The model under review builds one solid part; all positions refer to its coordinate system, in mm. Round coordinates to 2 decimals unless told otherwise and drop trailing zeros. Loops run counter-clockwise (first coordinate to the right, second up) from the corner with the lowest first, then second, coordinate; pieces in that order, holes last. Notation, with made-up numbers: (45, -36) -> (78, -36) arc R15 ccw to (78, -29) -> close; hole circle Ø10 at (29, 80). An arc over 180 degrees is marked (long way). Use a Markdown table: item, result. Add a question column.
1) Consider section D-D on z = 303. Give the boundary of the cut face in (x, y).
2) Consider section B-B on z = 212. Give the boundary of the cut face in (x, y), plus the area to 3 significant figures.
3) Consider section A-A on z = 277. Give the boundary of the cut face in (x, y), plus the area to 3 significant figures.
4) Consider section C-C on x = 9.5. Give the boundary of the cut face in (y, z).
5) Insertion check: pin 1 (1 mm diameter, centred on x = -31, y = 77.5, fed in from +Z); pin 2 (0.9 mm diameter, centred on y = 77, z = 316.5, fed in from -X); pin 3 (1.5 mm diameter, centred on y = 76, z = 316.5, fed in from +X); pin 4 (3 mm diameter, centred on x = 35, z = 303, fed in from -Y) (3 decimals). Each pin has a flat end and moves straight along its axis. Give the tip position at first contact, or say it passes through.
6) Wall thickness on probe 1 along X at (y, z) = (75.7, 303); probe 2 along Z at (x, y) = (35, 75.7); probe 3 along X at (y, z) = (76.5, 212): over which ranges is each line inside the solid? List them lowest first.
from build123d import *

# Parameters (mm, degrees)
PAD098_DEPTH    = 3
POCKET028_DEPTH = 3.001
SKETCH185_R     = 1.6
SKETCH185_W     = 50
SKETCH185_H     = 69.2
POCKET029_DEPTH = 3.001
SKETCH209_W     = 50.2
SKETCH209_H     = 87.2
POCKET043_DEPTH = 5
CHAMFER073_SIZE = 1
SKETCH214_R     = 1.6
POCKET046_DEPTH = 3.001


with BuildPart() as part:
    # Sketch183 → Pad098 (new body)
    with BuildSketch(Plane(origin=(0, 0, 0), x_dir=(-1, 0, 0), z_dir=(0, 1, 0))):
        Polygon((-40, 310), (-30, 310), (-30, 320), (30, 320), (30, 310), (40, 310), (40, 207), (-40, 207), align=None)
    extrude(amount=PAD098_DEPTH)

    # Sketch184 → Pocket028 (cut, through all)
    with BuildSketch(Plane(origin=(0, 0, 0), x_dir=(-1, 0, 0), z_dir=(0, 1, 0))):
        with BuildLine():
            ThreePointArc((-40, 294), (-44, 290), (-40, 286))
            Line((-40, 286), (-35, 286))
            ThreePointArc((-35, 286), (-31, 290), (-35, 294))
            Line((-35, 294), (-40, 294))
        make_face()
        with BuildLine():
            ThreePointArc((-40, 231), (-44, 227), (-40, 223))
            Line((-40, 223), (-35, 223))
            ThreePointArc((-35, 223), (-31, 227), (-35, 231))
            Line((-35, 231), (-40, 231))
        make_face()
        with BuildLine():
            ThreePointArc((40, 223), (44, 227), (40, 231))
            Line((40, 231), (35, 231))
            ThreePointArc((35, 231), (31, 227), (35, 223))
            Line((35, 223), (40, 223))
        make_face()
        with BuildLine():
            ThreePointArc((40, 286), (44, 290), (40, 294))
            Line((40, 294), (35, 294))
            ThreePointArc((35, 294), (31, 290), (35, 286))
            Line((35, 286), (40, 286))
        make_face()
    extrude(amount=POCKET028_DEPTH, mode=Mode.SUBTRACT)

    # Sketch185 (on Face5 of Pocket028) → Pocket029 (cut, through all)
    with BuildSketch(Plane(origin=(0, 3, 0), x_dir=(-1, 0, 0), z_dir=(0, 1, 0))):
        with Locations((22, 217.92)):
            Circle(SKETCH185_R)
        with Locations((-22, 217.92)):
            Circle(SKETCH185_R)
        with Locations((-22, 294)):
            Circle(SKETCH185_R)
        with Locations((22, 294)):
            Circle(SKETCH185_R)
        with Locations((0, 256)):
            Rectangle(SKETCH185_W, SKETCH185_H)
    extrude(amount=-POCKET029_DEPTH, mode=Mode.SUBTRACT)

    # Sketch209 (on Face5 of Pocket029) → Pocket043 (cut)
    with BuildSketch(Plane(origin=(0, 3, 0), x_dir=(-1, 0, 0), z_dir=(0, 1, 0))):
        with Locations((0, 254)):
            Rectangle(SKETCH209_W, SKETCH209_H)
    extrude(amount=-POCKET043_DEPTH, mode=Mode.SUBTRACT)

    # Chamfer073
    chamfer073_edges = [part.edges().sort_by_distance(p)[0] for p in [
        (-30, 1.5, 320),
        (-40, 1.5, 310),
        (-40, 1.5, 294),
        (-40, 1.5, 286),
        (-40, 1.5, 223),
        (-40, 1.5, 231),
        (-40, 1.5, 207),
        (40, 1.5, 207),
        (40, 1.5, 223),
        (40, 1.5, 231),
        (40, 1.5, 294),
        (40, 1.5, 286),
        (40, 1.5, 310),
        (30, 1.5, 320),
    ]]
    chamfer(chamfer073_edges, length=CHAMFER073_SIZE)

    # Sketch214 (on Face5 of Chamfer073) → Pocket046 (cut, through all)
    with BuildSketch(Plane(origin=(0, 3, 0), x_dir=(-1, 0, 0), z_dir=(0, 1, 0))):
        with Locations((35, 212)):
            Circle(SKETCH214_R)
        with Locations((-35, 212)):
            Circle(SKETCH214_R)
        with Locations((-35, 303)):
            Circle(SKETCH214_R)
        with Locations((35, 303)):
            Circle(SKETCH214_R)
    extrude(amount=-POCKET046_DEPTH, mode=Mode.SUBTRACT)


with BuildPart() as part_1:
    # Body086 placement: moved
    add(part.part.moved(Location((0, 75, 0))))


solid = part_1.part
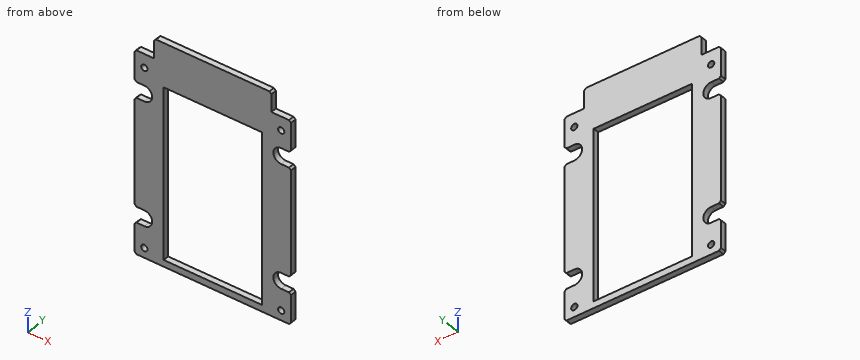
Result set:
| question | item | result |
|---|---|---|
| 1 | outline | (-40, 75) -> (-36.6, 75) -> (-36.6, 78) -> (-40, 78) -> close; (-33.4, 75) -> (33.4, 75) -> (33.4, 78) -> (-33.4, 78) -> close; (36.6, 75) -> (40, 75) -> (40, 78) -> (36.6, 78) -> close |
| 2 | outline | (-40, 75) -> (-36.6, 75) -> (-36.6, 78) -> (-40, 78) -> close; (-33.4, 75) -> (-25.1, 75) -> (-25.1, 78) -> (-33.4, 78) -> close; (25.1, 75) -> (33.4, 75) -> (33.4, 78) -> (25.1, 78) -> close; (36.6, 75) -> (40, 75) -> (40, 78) -> (36.6, 78) -> close |
| 2 | area | 70.2 mm2 |
| 3 | outline | (-40, 75) -> (-25.1, 75) -> (-25.1, 78) -> (-40, 78) -> close; (25.1, 75) -> (40, 75) -> (40, 78) -> (25.1, 78) -> close |
| 3 | area | 89.4 mm2 |
| 4 | outline | (75, 207) -> (78, 207) -> (78, 210.4) -> (75, 210.4) -> close; (75, 297.6) -> (78, 297.6) -> (78, 320) -> (75, 320) -> close |
| 5 | pin 1 | z = 310 |
| 5 | pin 2 | x = -30 |
| 5 | pin 3 | x = 30 |
| 5 | pin 4 | through |
| 6 | probe 1 | -40 to -36.6, -33.4 to 33.4, 36.6 to 40 |
| 6 | probe 2 | 207 to 210.4, 213.6 to 223, 231 to 286, 294 to 301.4, 304.6 to 310 |
| 6 | probe 3 | -40 to -36.6, -33.4 to -25.1, 25.1 to 33.4, 36.6 to 40 |
